Verification items for the finished model (mm, model axes). Round coordinates to 2 decimals unless told otherwise and drop trailing zeros. Write each loop counter-clockwise with the first axis right and the second up, starting at its lowest first coordinate (ties: lowest second). Pieces come first, ordered by that corner, then holes. Notation, with made-up numbers: (63.25, 13.5) -> (104.25, 13.5) arc R20 ccw to (104.25, 50.5) -> close; hole circle Ø6 at (48.25, 72). An arc over 180 degrees is marked (long way). Use CSV: the item, a comma, the result in double quotes.
```python
from build123d import *

# Parameters (mm, degrees)
EXTRUDE_1_DEPTH             = 3
HOLE_WIZARD_1_AT_2_COUNT    = 2
HOLE_WIZARD_1_AT_2_PITCH    = 280
HOLE_WIZARD_1_AT_3_COUNT    = 2
HOLE_WIZARD_1_AT_3_PITCH    = 395.979797464
HOLE_WIZARD_1_AT_4_COUNT    = 2
HOLE_WIZARD_1_AT_4_PITCH    = 280
SKETCH_4_W                  = 8
SKETCH_4_H                  = 15
EXTRUDE_2_DEPTH             = 1
HOLE_WIZARD_1_2_D           = 3.4
HOLE_WIZARD_1_2_CSINK_D     = 6.6
HOLE_WIZARD_1_2_CSINK_ANGLE = 90


with BuildPart() as part:
    # 草图1 → 凸台-拉伸1 (new body)
    with BuildSketch(Plane.XY):
        with BuildLine():
            Line((-147, 155), (147, 155))
            ThreePointArc((147, 155), (152.656854249, 152.656854249), (155, 147))
            Line((155, 147), (155, -147))
            ThreePointArc((155, -147), (152.656854249, -152.656854249), (147, -155))
            Line((147, -155), (-147, -155))
            ThreePointArc((-147, -155), (-152.656854249, -152.656854249), (-155, -147))
            Line((-155, -147), (-155, 147))
            ThreePointArc((-155, 147), (-152.656854249, 152.656854249), (-147, 155))
        make_face()
    extrude(amount=EXTRUDE_1_DEPTH)

    # 草图2 → Hole Wizard 1 (revolve, cut)
    with BuildSketch(Plane(origin=(-140, 140, 3), x_dir=(0, -1, 0), z_dir=(1, 0, 0))):
        Polygon((0, 0), (0, 3), (2.25, 3), (2.25, 2.75), (5, 0), align=None)
    hole_wizard_1 = revolve(axis=Axis((-140, 140, 9.35), (0, 0, -1)), mode=Mode.SUBTRACT)

    # Hole Wizard 1 at 2: Hole Wizard 1 ×2
    with Locations(*[(i * HOLE_WIZARD_1_AT_2_PITCH, 0, 0) for i in range(1, HOLE_WIZARD_1_AT_2_COUNT)]):
        add(hole_wizard_1, mode=Mode.SUBTRACT)

    # Hole Wizard 1 at 3: Hole Wizard 1 ×2
    with Locations(*[Vector(0.707106781, -0.707106781, 0) * (i * HOLE_WIZARD_1_AT_3_PITCH) for i in range(1, HOLE_WIZARD_1_AT_3_COUNT)]):
        add(hole_wizard_1, mode=Mode.SUBTRACT)

    # Hole Wizard 1 at 4: Hole Wizard 1 ×2
    with Locations(*[(0, -i * HOLE_WIZARD_1_AT_4_PITCH, 0) for i in range(1, HOLE_WIZARD_1_AT_4_COUNT)]):
        add(hole_wizard_1, mode=Mode.SUBTRACT)

    # 草图4 → 凸台-拉伸2 (add)
    with BuildSketch(Plane(origin=(0, 0, 0), x_dir=(-1, 0, 0), z_dir=(0, 0, -1))):
        with Locations((-19, 111.5)):
            Rectangle(SKETCH_4_W, SKETCH_4_H)
        with Locations((-33, 111.5)):
            Rectangle(SKETCH_4_W, SKETCH_4_H)
    extrude(amount=EXTRUDE_2_DEPTH)

    # Hole Wizard 1 2 (through all)
    with Locations(Plane.XY.offset(3)):
        with Locations((150, -105), (150, 105), (-150, 105), (-150, -105)):
            CounterSinkHole(HOLE_WIZARD_1_2_D / 2, HOLE_WIZARD_1_2_CSINK_D / 2, counter_sink_angle=HOLE_WIZARD_1_2_CSINK_ANGLE)


solid = part.part
```
Q1. Mould release check, pull along Y, two halves, no side actions. Record for faces 1 (the conical face through (-140.73, 137.69, 0.42)), 2 (the flat face through (19, 112, -1)), 3 (the conical face through (-140.73, -142.31, 0.42)), 4 (the cylindrical face through (152.719, -152.594, 1.479)): released by +Y, released by -Y, zero draft, split by the parting line, or undercut.
Filled in:
face 1,"undercut"
face 2,"zero draft"
face 3,"undercut"
face 4,"released by -Y"
Q2. Go/stop test with flat-tipped pins: P1, Ø5, axis at x = -140, y = -140, coming from the -Z side; P2, Ø0.5, axis at x = 31.5, z = -0.5, coming from the -Y side; P3, Ø3.5, axis at x = 140, y = -140, coming from the +Z side; P4, Ø0.5, axis at y = 109.5, z = -0.5, coming from the +X side. Record where each tip stops, or that it passes through.
Filled in:
P1,"z = 0"
P2,"y = 104"
P3,"through"
P4,"x = 37"
Q3. Material ranges on L1, parallel to X at y = -105, z = 0.5; L2, parallel to Y at x = 140, z = 0.15; L3, parallel to Y at x = -150, z = 1, recorded low to high.
Filled in:
L1,"-155 to -151.7, -148.3 to 148.3, 151.7 to 155"
L2,"-155 to -142.25, -137.75 to 137.75, 142.25 to 155"
L3,"-154.42 to -106.7, -103.3 to 103.3, 106.7 to 154.42"
Q4. Section check A-A (y = -113). Record the cut outline in (x, z).
Filled in:
outline,"(-155, 0) -> (155, 0) -> (155, 3) -> (-155, 3) -> close"
